Here's the drawing with two shaded views (mm, measured from the low corner). I have some questions. A direction names the side the tool comes from. Coordinates: 2 decimals unless noted, no trailing zeros. Loops run counter-clockwise (first coordinate to the right, second up) from the corner with the lowest first, then second, coordinate; pieces in that order, holes last. Notation, with made-up numbers: (55, -32.75) - (86, -32.75) arc R18 ccw to (86, -25.75) - close; hole circle Ø4 at (87.25, 60.25). An arc over 180 degrees is marked (long way). Use a Markdown table: item, result.
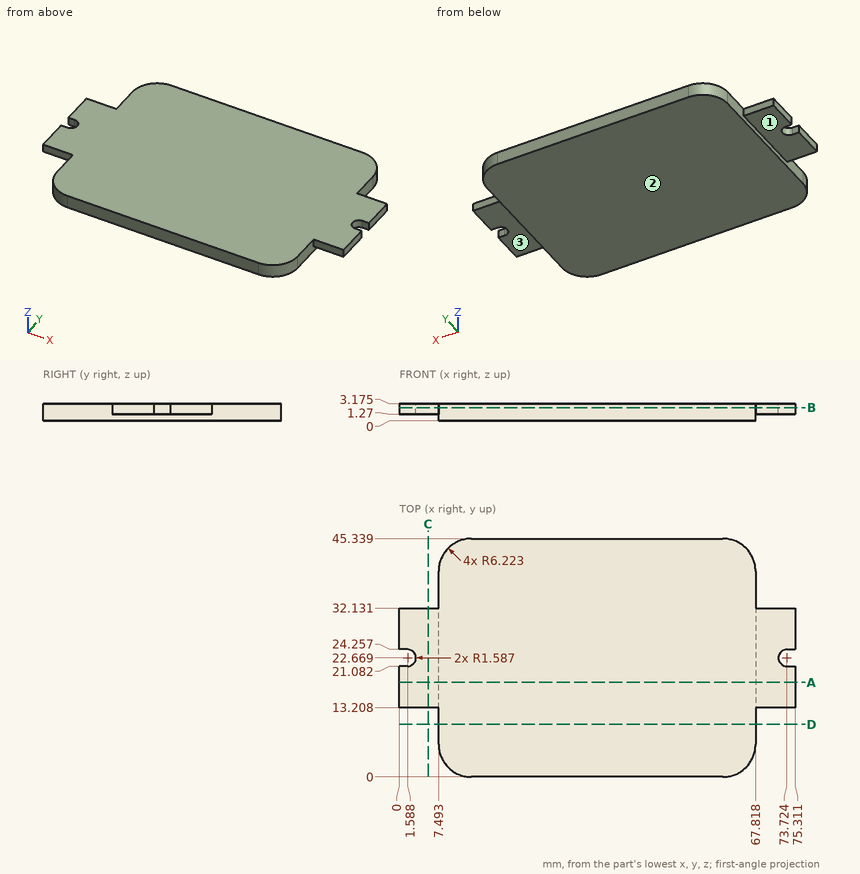
Q1. I want a section at A-A, the plane y = 18. Write out the boundary of the cut face in (x, z) (1 decimal).
Check values:
| item | result |
|---|---|
| outline | (0, 1.3) - (7.5, 1.3) - (7.5, 0) - (67.8, 0) - (67.8, 1.3) - (75.3, 1.3) - (75.3, 3.2) - (0, 3.2) - close |
Q2. I want a section at D-D, the plane y = 10. Write out the boundary of the cut face in (x, z) (1 decimal).
Check values:
| item | result |
|---|---|
| outline | (7.5, 0) - (67.8, 0) - (67.8, 3.2) - (7.5, 3.2) - close |
Q3. I want a section at B-B, the plane z = 2.5. Write out the boundary of the cut face in (x, y) (1 decimal).
Check values:
| item | result |
|---|---|
| outline | (0, 13.2) - (7.5, 13.2) - (7.5, 6.2) arc R6.2 ccw to (13.7, 0) - (61.6, 0) arc R6.2 ccw to (67.8, 6.2) - (67.8, 13.2) - (75.3, 13.2) - (75.3, 21.1) - (73.7, 21.1) arc R1.6 cw to (73.7, 24.3) - (75.3, 24.3) - (75.3, 32.1) - (67.8, 32.1) - (67.8, 39.1) arc R6.2 ccw to (61.6, 45.3) - (13.7, 45.3) arc R6.2 ccw to (7.5, 39.1) - (7.5, 32.1) - (0, 32.1) - (0, 24.3) - (1.6, 24.3) arc R1.6 cw to (1.6, 21.1) - (0, 21.1) - close |
Q4. Please list where these lines run through material, in increasing order: L1, parallel to X at y = 35, z = 2.9; L2, parallel to Y at x = 4, z = 2.85; L3, parallel to Y at x = 72.5, z = 2.8 (1 decimal). Write a range as from..to.
Check values:
| item | result |
|---|---|
| L1 | 7.49..67.82 |
| L2 | 13.21..32.13 |
| L3 | 13.2..21.7, 23.7..32.1 |
Q5. Will these pins go through, and if not, where does the flat tip stop? P1, Ø8, axis at x = 73, y = 27, coming from the -Z side; P2, Ø1.6, axis at y = 30, z = 1, coming from the -X side; P3, Ø1, axis at x = 72.5, z = 2.5, coming from the -Y side; P4, Ø0.5, axis at x = 0.5, z = 2, coming from the +Y side.
Check values:
| item | result |
|---|---|
| P1 | z = 1.27 |
| P2 | x = 0 |
| P3 | y = 13.21 |
| P4 | y = 32.13 |
Q6. I want a section at C-C, the plane x = 5.5. Write out the boundary of the cut face in (y, z) (1 decimal).
Check values:
| item | result |
|---|---|
| outline | (13.2, 1.3) - (32.1, 1.3) - (32.1, 3.2) - (13.2, 3.2) - close |
Q7. Which directions (+Z, -Z, +X, -X, +Y, -Y) give clear straight access to the entire face, cutting with the end or side of a thin tool? Please do the marked faces 1, 2 and 3.
Check values:
| item | result |
|---|---|
| face 1 | -Z, -X, +Y, -Y |
| face 2 | -Z, +X, -X, +Y, -Y |
| face 3 | -Z, +X, +Y, -Y |
